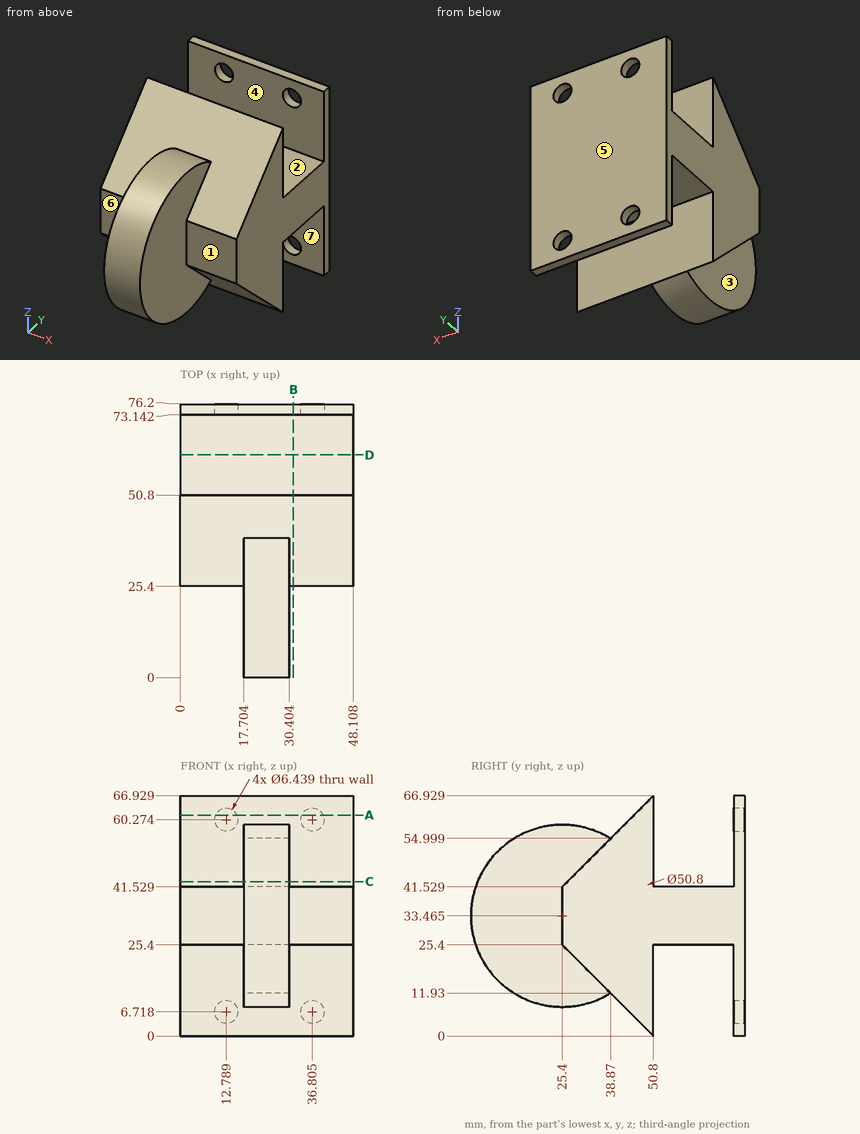
Here's the drawing with two shaded views (mm, measured from the low corner). I have some questions. A direction names the side the tool comes from. Coordinates: 2 decimals unless noted, no trailing zeros. Write each loop counter-clockwise with the first axis right and the second up, starting at its lowest first coordinate (ties: lowest second). Pieces come first, ordered by that corner, then holes.
Item 1: If I drill on line 1 (Z direction, x = 28.5, y = 72); line 2 (Y direction, x = 35.5, z = 24.5) (1 decimal); line 3 (Y direction, x = 33, z = 52.5) (1 decimal), over which ranges is the centre line in solid material (lowest first)?
Item 2: I want a section at B-B on x = 31.5. Write out the boundary of the cut face in (y, z).
Item 3: I want a section at C-C on z = 43. Write out the boundary of the cut face in (x, y), and give its area (3 significant figures).
Item 4: If we mould it in two halves opening along Y, with no side actions, what happens to the marked faces 1, 2 and 3? For each: +Y half, -Y half, draft (parallel to the pull), parting line (faces both ways), or undercut.
Item 5: Will these pins go through, and if not, where does the flat tip stop? pin 1 (2 mm diameter, centred on x = 27, y = 44.5, fed in from +Z); pin 2 (5 mm diameter, centred on y = 41.5, z = 11, fed in from -X); pin 3 (1.5 mm diameter, centred on x = 36, y = 38.5, fed in from -Z); pin 4 (6.5 mm diameter, centred on x = 29, y = 57, fed in from +Z).
Item 6: I want a section at A-A on z = 61.5. Write out the boundary of the cut face in (x, y) (1 decimal).
Item 7: I want a section at D-D on y = 62. Write out the boundary of the cut face in (x, z).
Item 8: On a 3-axis mill with a long thin cutter (end or side, diameter ignored), from which of +Z, -Z, +X, -X, +Y, -Y can I reach the whole of each face in a straight line? I mean the marked faces 4, 5, 6 and 7. Say none if no direction works.
Findings below:
1. line 1: z = 25.4 to 41.53
1. line 2: y = 26.3 to 50.8, 73.1 to 76.2
1. line 3: y = 36.4 to 50.8, 73.1 to 76.2
2. outline: (25.4, 25.4) - (50.8, 0) - (50.8, 25.4) - (73.14, 25.4) - (73.14, 0) - (76.2, 0) - (76.2, 66.93) - (73.14, 66.93) - (73.14, 41.53) - (50.8, 41.53) - (50.8, 66.93) - (25.4, 41.53) - close
3. outline: (0, 26.87) - (17.7, 26.87) - (17.7, 1.86) - (30.4, 1.86) - (30.4, 26.87) - (48.11, 26.87) - (48.11, 50.8) - (0, 50.8) - close; (0, 73.14) - (48.11, 73.14) - (48.11, 76.2) - (0, 76.2) - close
3. area: 1,620 mm2
4. face 1: -Y half
4. face 2: undercut
4. face 3: draft
5. pin 1: stops at z = 61.63
5. pin 2: stops at x = 0
5. pin 3: stops at z = 11.55
5. pin 4: stops at z = 41.53
6. outline: (0, 45.4) - (48.1, 45.4) - (48.1, 50.8) - (0, 50.8) - close; (0, 73.1) - (9.8, 73.1) - (9.8, 76.2) - (0, 76.2) - close; (15.8, 73.1) - (33.8, 73.1) - (33.8, 76.2) - (15.8, 76.2) - close; (39.8, 73.1) - (48.1, 73.1) - (48.1, 76.2) - (39.8, 76.2) - close
7. outline: (0, 25.4) - (48.11, 25.4) - (48.11, 41.53) - (0, 41.53) - close
8. face 4: +Z, +X, -X
8. face 5: +Z, -Z, +X, -X, +Y
8. face 6: +Z, -Z, -X, -Y
8. face 7: -Z, +X, -X
